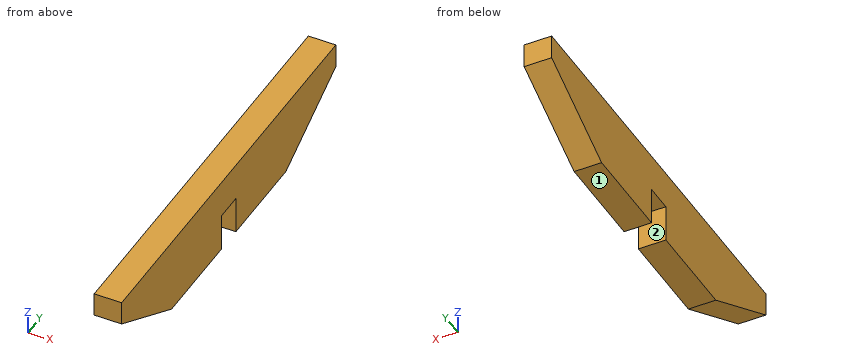
```python
from build123d import *

# Parameters (mm, degrees)
F0_W     = 50.8
F0_H     = 69.85
F1_DEPTH = 50.8


with BuildPart() as f1:
    # F0 (on Right) → F1 (new body)
    with BuildSketch(Plane.YZ):
        Polygon((-177.8, -27.121778), (0, -27.121778), (0, 42.728222), (0, 112.578222), (-355.6, 112.578222), (-355.6, 67.942142), align=None)
        with Locations((25.4, 77.653222)):
            Rectangle(F0_W, F0_H)
        Polygon((50.8, 112.578222), (50.8, 42.728222), (50.8, -27.121778), (228.6, -27.121778), (406.4, 66.987783), (406.4, 112.578222), align=None)
    extrude(amount=F1_DEPTH)


solid = f1.part
```
The listing builds one solid part. Answer for the finished solid, in the listing's coordinates (mm). Face numbers are marked on the shaded views. A direction names the side the tool comes from. Coordinates: 2 decimals unless noted, no trailing zeros. Loops run counter-clockwise (first coordinate to the right, second up) from the corner with the lowest first, then second, coordinate; pieces in that order, holes last. Notation, with made-up numbers: M -7.5,52.5 L 41.5,52.5 A14 cw 41.5,61.5 Z; hole C 2.25,32.5 d11. An arc over 180 degrees is marked long. Answer as a JSON object with one key per item and string values. Group by question number.
Item 1: Which of the six approach directions +Z, -Z, +X, -X, +Y, -Y give full straight-line access (tool end or side, diameter ignored) to the marked faces 1 and 2?
Item 2: Section B-B (z = 8) is taken. Write down the section's boundary in (x, y), and give its area (3 significant figures).
Item 3: Section C-C (y = 23) is taken. Write down the section's boundary in (x, z).
Item 4: Section A-A (x = 11.5) is taken. Write down the section's boundary in (y, z), and give its area (3 significant figures).
Item 5: Section D-D (z = 36.5) is taken. Write down the section's boundary in (x, y).
Item 6: Each of these flat-tipped pins is pushed along its axis until it touches: P1, Ø4, axis at x = 23.5, z = 6.5, coming from the +Y side; P2, Ø1, axis at x = 33.5, z = 58.5, coming from the -Y side; P3, Ø12, axis at x = 40.5, z = 9.5, coming from the -Y side. Where does it stop, or does it pass through?
Item 7: Consider L1, parallel to Y at x = 44, z = 31; L2, parallel to Y at x = 5, z = 30; L3, parallel to Z at x = 35.5, y = 30. Determine where each line is inside the solid, lowest interval first.
Solved:
{
 "1": {"face 1": "-Z, +X, -X, +Y, -Y", "face 2": "-Z, +X, -X"},
 "2": {"outline": "M 0,-243.49 L 50.8,-243.49 L 50.8,0 L 0,0 Z; M 0,50.8 L 50.8,50.8 L 50.8,294.96 L 0,294.96 Z", "area": "24,800 mm2"},
 "3": {"outline": "M 0,42.73 L 50.8,42.73 L 50.8,112.58 L 0,112.58 Z"},
 "4": {"outline": "M -355.6,67.94 L -177.8,-27.12 L 0,-27.12 L 0,42.73 L 50.8,42.73 L 50.8,-27.12 L 228.6,-27.12 L 406.4,66.99 L 406.4,112.58 L -355.6,112.58 Z", "area": "86,100 mm2"},
 "5": {"outline": "M 0,-296.79 L 50.8,-296.79 L 50.8,0 L 0,0 Z; M 0,50.8 L 50.8,50.8 L 50.8,348.8 L 0,348.8 Z"},
 "6": {"P1": "stops at y = 295.9", "P2": "stops at y = -338.88", "P3": "stops at y = -257.52"},
 "7": {"L1": "y = -286.51 to 0, 50.8 to 338.41", "L2": "y = -284.64 to 0, 50.8 to 336.52", "L3": "z = 42.73 to 112.58"}
}
